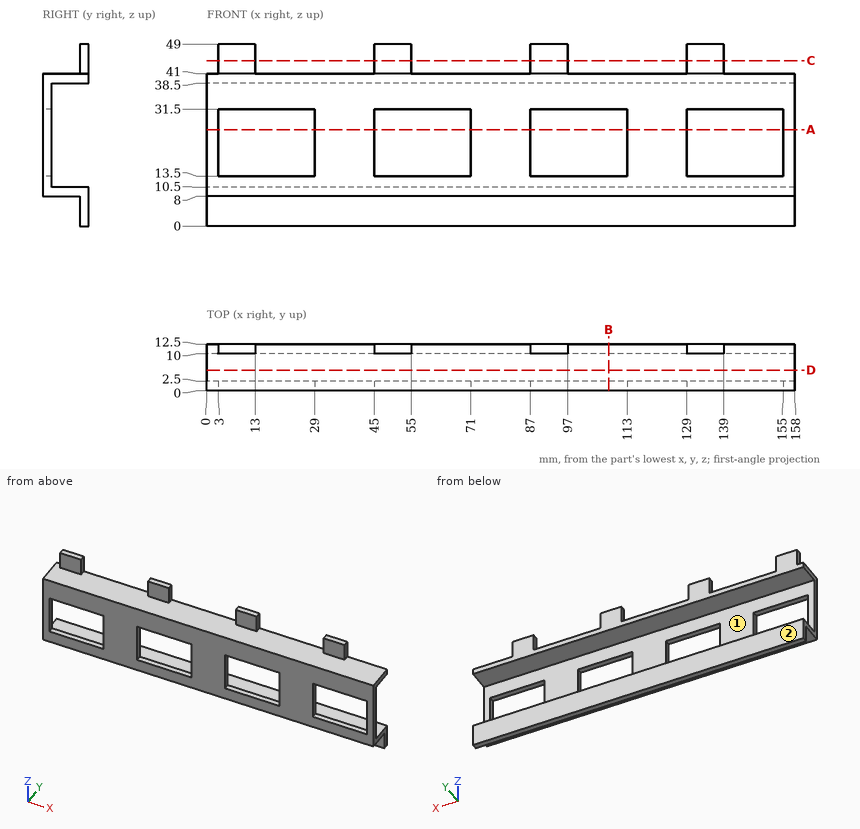
Study the drawing (mm; zero at the part's minimum x, y, z) and answer. A direction names the side the tool comes from. Give positions to 0.01 mm unless a question says otherwise; leave off trailing zeros. Loops run counter-clockwise (first coordinate to the right, second up) from the corner with the lowest first, then second, coordinate; pieces in that order, holes last. Notation, with made-up numbers: (-0.75, -36) - (38.25, -36) arc R35 ccw to (38.25, 2) - close; hole circle Ø9 at (70.5, 76). An arc over 180 degrees is marked (long way). One line per question, with ' | ' between items.
(1) The part is cut by section A-A (z = 26). Write down the section's boundary in (x, y), then the cut area to 3 significant figures.
Recorded:
outline: (0, 0) - (3, 0) - (3, 2.5) - (0, 2.5) - close; (29, 0) - (45, 0) - (45, 2.5) - (29, 2.5) - close; (71, 0) - (87, 0) - (87, 2.5) - (71, 2.5) - close; (113, 0) - (129, 0) - (129, 2.5) - (113, 2.5) - close; (155, 0) - (158, 0) - (158, 2.5) - (155, 2.5) - close | area: 135 mm²
(2) A tool of negligible diameter and unlimited length cuts with its end or side. For the marked faces 1 and 2, from which of +Z, -Z, +X, -X, +Y, -Y can it reach the whole face along a straight path? Write none if from no direction.
Recorded:
face 1: +X, -X, +Y | face 2: +Z, -Z, +X, -X, +Y
(3) Each of these flat-tipped pins is pushed along its axis until it touches: pin 1 Ø6.5 at (x, z) = (10.5, 46.5) entering from -Y; pin 2 Ø2 at (y, z) = (11, 43.5) entering from -X; pin 3 Ø1.2 at (y, z) = (11, 47) entering from +X. Where does it stop, or does it pass through?
Recorded:
pin 1: stops at y = 10 | pin 2: stops at x = 3 | pin 3: stops at x = 139
(4) The part is cut by section C-C (z = 44.5). Write down the section's boundary in (x, y).
Recorded:
outline: (3, 10) - (13, 10) - (13, 12.5) - (3, 12.5) - close; (45, 10) - (55, 10) - (55, 12.5) - (45, 12.5) - close; (87, 10) - (97, 10) - (97, 12.5) - (87, 12.5) - close; (129, 10) - (139, 10) - (139, 12.5) - (129, 12.5) - close
(5) The part is cut by section D-D (y = 5.5). Write down the section's boundary in (x, z), then the cut area to 3 significant figures.
Recorded:
outline: (0, 8) - (158, 8) - (158, 10.5) - (0, 10.5) - close; (0, 38.5) - (158, 38.5) - (158, 41) - (0, 41) - close | area: 790 mm²
(6) Straight lines are drawn through the part: probe 1 along X at (y, z) = (1.5, 23.5); probe 2 along Z at (x, y) = (91.5, 3.5); probe 3 along Z at (x, y) = (134.5, 10.75). For each, find the intervals that lie inside material, in ascending order.
Recorded:
probe 1: x = 0 to 3, 29 to 45, 71 to 87, 113 to 129, 155 to 158 | probe 2: z = 8 to 10.5, 38.5 to 41 | probe 3: z = 0 to 10.5, 38.5 to 49
(7) The part is cut by section B-B (x = 108). Write down the section's boundary in (y, z), then the cut area to 4 significant figures.
Recorded:
outline: (0, 8) - (10, 8) - (10, 0) - (12.5, 0) - (12.5, 10.5) - (2.5, 10.5) - (2.5, 13.5) - (0, 13.5) - close; (0, 31.5) - (2.5, 31.5) - (2.5, 38.5) - (12.5, 38.5) - (12.5, 41) - (0, 41) - close | area: 107.5 mm²
